Can you work these out from the drawing? Everything is in mm from the part's minimum corner. A direction names the side the tool comes from. Round coordinates to 2 decimals unless told otherwise and drop trailing zeros. Write each loop counter-clockwise with the first axis right and the second up, starting at its lowest first coordinate (ties: lowest second). Pieces come first, ordered by that corner, then holes. Notation, with made-up numbers: (-25, -33) - (6, -33) arc R25 ccw to (6, -14) - close; hole circle Ø1 at (-24, 26.25). An arc over 180 degrees is marked (long way). One line per item, written item: value. Start each with the question number.
Item 1: If I drill on line 1 (Z direction, x = 18, y = 29); line 2 (Y direction, x = 18, z = 49); line 3 (Z direction, x = 20.5, y = 24), over which ranges is the centre line in solid material (lowest first)?
Item 2: Imagine slicing it at A-A, the plane x = 17.5. Please give me the cut outline in (y, z).
Item 3: Imagine slicing it at C-C, the plane z = 63. Please give me the cut outline in (x, y).
Item 4: Imagine slicing it at D-D, the plane z = 26. Please give me the cut outline in (x, y).
Item 5: For the marked faces 1, 2 and 3, which set-ups out of +Z, -Z, +X, -X, +Y, -Y let a thin tool reach every point of the face, with its end or its side?
Item 6: For P1, Ø3, axis at y = 28, z = 33, coming from the -X side; P2, Ø16.5, axis at x = 19.5, y = 10.5, coming from the +Z side; P3, Ø2, axis at y = 24.5, z = 46.5, coming from the -X side; P4, Ø1.5, axis at y = 24.5, z = 28, coming from the -X side, each with a flat end and sliding along its axis, tell me the tip position at first contact or that it passes through.
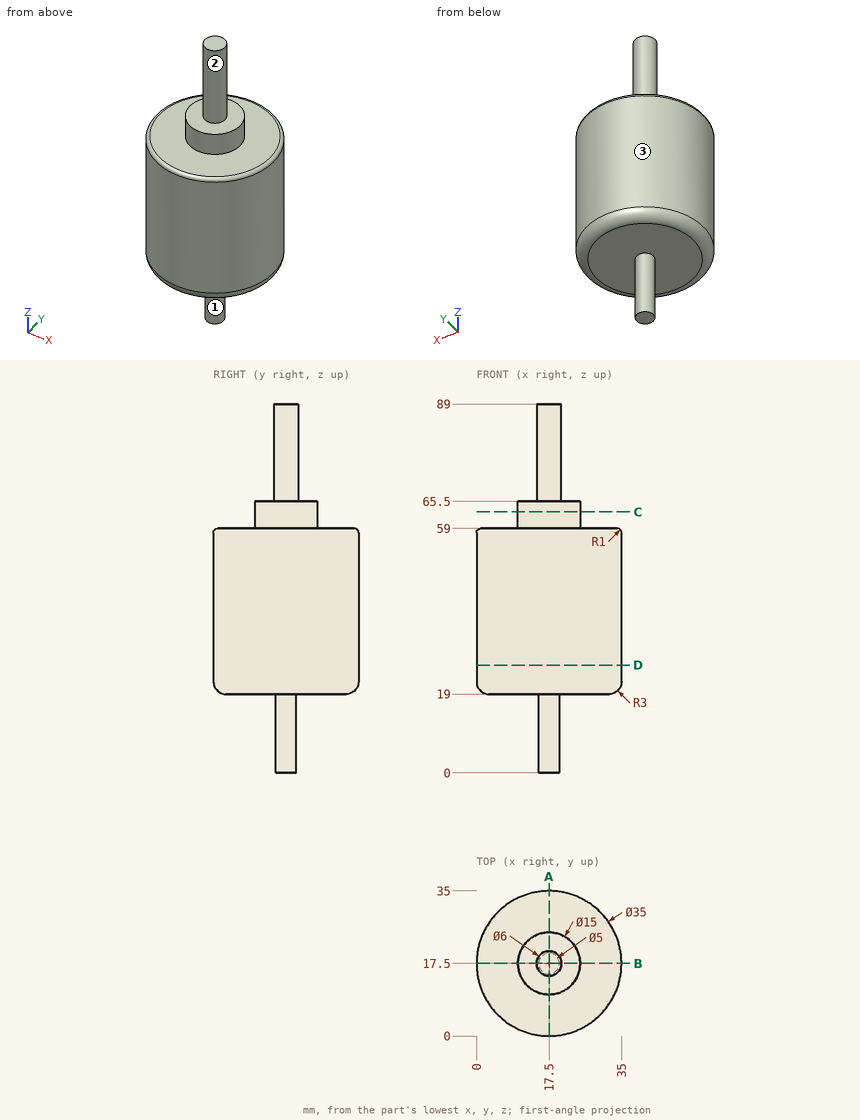
Values follow:
1. line 1: z = 19 to 59
1. line 2: y = 0.01 to 34.99
1. line 3: z = 19 to 65.5
2. outline: (0, 22) arc R3 ccw to (3, 19) - (15, 19) - (15, 0) - (20, 0) - (20, 19) - (32, 19) arc R3 ccw to (35, 22) - (35, 58) arc R1 ccw to (34, 59) - (25, 59) - (25, 65.5) - (20.5, 65.5) - (20.5, 89) - (14.5, 89) - (14.5, 65.5) - (10, 65.5) - (10, 59) - (1, 59) arc R1 ccw to (0, 58) - close
3. outline: circle Ø15 at (17.5, 17.5)
4. outline: circle Ø35 at (17.5, 17.5)
5. face 1: -Z
5. face 2: +Z
5. face 3: +Z, -Z
6. P1: stops at x = 2.49
6. P2: stops at z = 89
6. P3: stops at x = 1.06
6. P4: stops at x = 1.15
